Answer from the drawing. Dimensions are ordinates in mm from the lowest x, y and z of the part. Give positions to 0.01 mm unless a question says otherwise; leave off trailing zeros. Write each loop counter-clockwise with the first axis right and the second up, starting at its lowest first coordinate (ties: lowest second). Pieces come first, ordered by that corner, then holes.
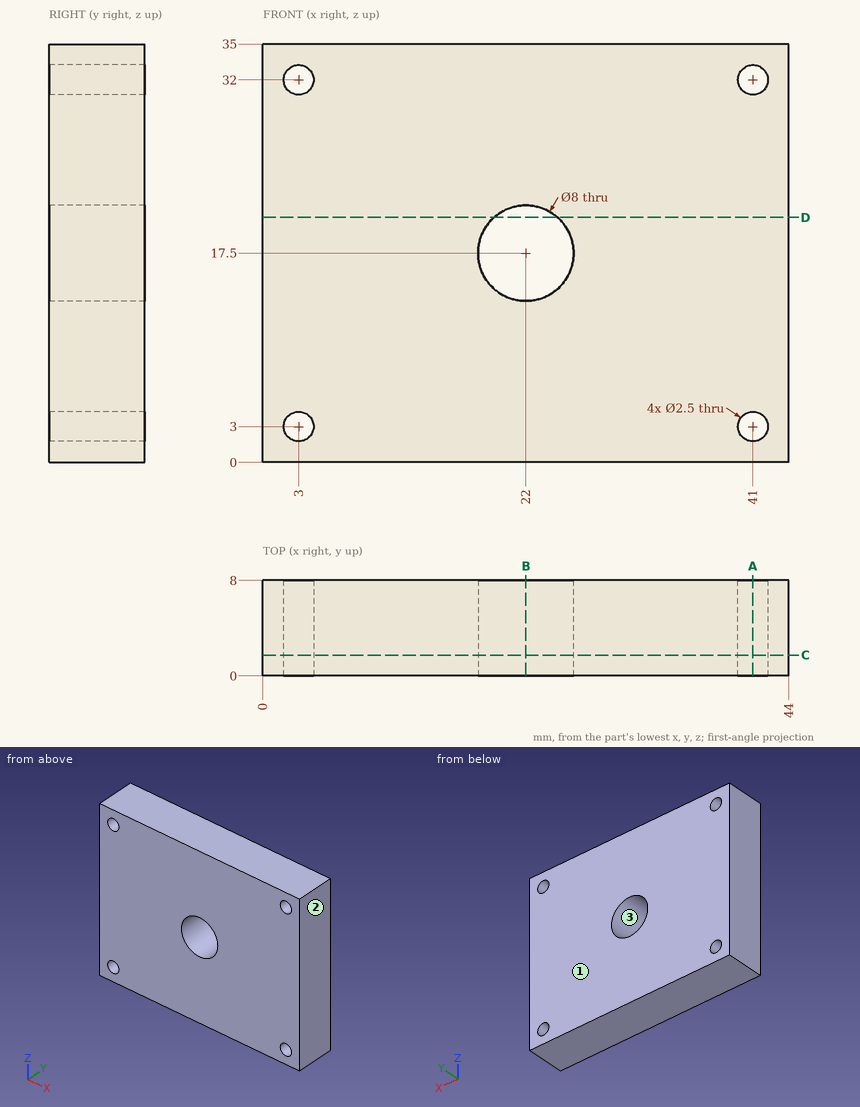
Item 1: A cutting plane is placed at A-A, the plane x = 41. Give the vertices of the cut face in (y, z), plus the area to 3 significant figures.
Conclusion:
outline: (0, 0) - (8, 0) - (8, 1.75) - (0, 1.75) - close; (0, 4.25) - (8, 4.25) - (8, 30.75) - (0, 30.75) - close; (0, 33.25) - (8, 33.25) - (8, 35) - (0, 35) - close
area: 240 mm2
Item 2: A cutting plane is placed at C-C, the plane y = 1.75. Give the vertices of the cut face in (x, z).
Conclusion:
outline: (0, 0) - (44, 0) - (44, 35) - (0, 35) - close; hole circle Ø2.5 at (3, 3); hole circle Ø2.5 at (3, 32); hole circle Ø8 at (22, 17.5); hole circle Ø2.5 at (41, 3); hole circle Ø2.5 at (41, 32)
Item 3: A cutting plane is placed at B-B, the plane x = 22. Give the vertices of the cut face in (y, z), plus the area to 3 significant figures.
Conclusion:
outline: (0, 0) - (8, 0) - (8, 13.5) - (0, 13.5) - close; (0, 21.5) - (8, 21.5) - (8, 35) - (0, 35) - close
area: 216 mm2
Item 4: Each of these flat-tipped pins is pushed along its axis until it touches: P1, Ø1.5, axis at x = 22, z = 21, coming from the -Y side; P2, Ø2, axis at x = 41, z = 32, coming from the -Y side. Where does it stop, or does it pass through?
Conclusion:
P1: stops at y = 0
P2: passes through
Item 5: Consider probe 1 along X at (y, z) = (2.5, 32); probe 2 along Z at (x, y) = (3, 2.25); probe 3 along X at (y, z) = (2, 17.5). Determine where each line is inside the solid, lowest interval first.
Conclusion:
probe 1: x = 0 to 1.75, 4.25 to 39.75, 42.25 to 44
probe 2: z = 0 to 1.75, 4.25 to 30.75, 33.25 to 35
probe 3: x = 0 to 18, 26 to 44
Item 6: Determine the mould class of the marked faces 1, 2 and 3 for opening direction X: pulls with the +X half, pulls with the -X half, needs draft (parallel to the pull), parting line crosses it, or undercut.
Conclusion:
face 1: needs draft
face 2: pulls with the +X half
face 3: undercut
Item 7: A cutting plane is placed at D-D, the plane z = 20.5. Give the vertices of the cut face in (x, y).
Conclusion:
outline: (0, 0) - (19.35, 0) - (19.35, 8) - (0, 8) - close; (24.65, 0) - (44, 0) - (44, 8) - (24.65, 8) - close
